Autodesk Inventor part; units mm, degrees
ref_plane "Work Plane1" through (30.1625, 0, 0) normal (0, 0, -1) x (1, 0, 0)
ref_plane "YZ Plane" through (0, 0, 0) normal (1, 0, 0) x (0, 1, 0)
ref_plane "XZ Plane" through (0, 0, 0) normal (0, 1, 0) x (-1, 0, 0)
sketch "Эскиз1" plane through (0, 0, 0) normal (0, 0, 1) x (1, 0, 0)
  line L0 (-6, 0) -> (25, 0)
  line L1 (25, 0) -> (25, 5)
  line L2 (25, 5) -> (1.5, 5)
  line L3 (1.5, 5) -> (0.5798, 5)
  line L4 (0.5798, 5) -> (0, 5)
  line L5 (0, 5) -> (0, 8)
  line L6 (-12.2, 0) -> (31.2, 0)
  line L7 (0, -1.6) -> (0, 9.6)
  line L8 (-6, 0) -> (-6, 8)
  line L9 (0, 8) -> (-6, 8)
  dimension "d0" = 25
  dimension "d1" = 23.5
  dimension "d2" = 0.9202
  dimension "d3" = 6
  dimension "d4" = 10
  dimension "d5" = 10
  dimension "d9" = 16
  dimension "d10" = 0
revolve "Базовый элемент" add sketch "Эскиз1" angle 360 about axis through (-6, 0, 0) along (1, 0, 0)
sketch "Эскиз2" plane through (-6, 0, 0) normal (-1, 0, 0) x (0, 0, 1)
  circle A0 centre (0, 0) radius 8
  line L0 (0, 0) -> (0, 8)
  line L1 (-8, 1.05) -> (8, 1.05)
  line L2 (8, 1.05) -> (8, -1.05)
  line L3 (8, -1.05) -> (-8, -1.05)
  line L4 (-8, -1.05) -> (-8, 1.05)
  line L5 (-8, 0) -> (8, 0) construction
  line L6 (0, 1.05) -> (0, -1.05) construction
  dimension "d11" = 2.1
  dimension "d12" = 16
fillet "Сопряжение1" radius 0.01 1 edges at (-6, -8, 0)
extrude "Паз" cut sketch "Эскиз2" against normal blind 4.2 contours A0 L3 L1 | L2 L3 A0 | A0 L1 L2 | L3 L4 A0 | A0 L4 L1
thread "Резьба"
chamfer "Chamfer4" distance 1 angle 45 1 edges at (25, -5, 0)
ref_plane "Work Plane1" through (30.1625, 0, 0) normal (0, 0, -1) x (1, 0, 0)
equation "\"d11\" = SBR"
equation "\"d12\" = KOD"
equation "\"d13\" = RR"
equation "\"d16\" = STI"
equation "\"d14\" = GEL"
equation "\"d40\" = 0.1 * GD"
equation "\"d0\" = NLG"
equation "\"d1\" = GEL"
equation "\"d2\" = GAL"
equation "\"d3\" = KOH"
equation "\"d4\" = GD"
equation "\"d5\" = BDM"
equation "\"d9\" = KOD"
equation "\"GD\" = NND"
equation "\"NLG\" = 25"
equation "\"GEL\" = 23.5"
equation "\"KOD\" = 16"
equation "\"KOH\" = 6"
equation "\"GAL\" = 0.61345 * PTC"
equation "\"BDM\" = NND"
equation "\"RR\" = 0.01"
equation "\"SBR\" = 2.1"
equation "\"STI\" = 4.2"
equation "\"KEWI\" = 0"
equation "\"GUL\" = 0.61345 * PTC"
equation "\"SPD\" = NND - 1.2269 * PTC"
equation "\"PTC\" = 1.5"
equation "\"TOA\" = 30deg"
equation "\"FAWI\" = 45deg"
equation "\"GD1\" = THREADDIA - 1.2269 * PTC"
properties part number "Винт M10-6gx25 ГОСТ 1491-80" material "Сталь, мягкая"
Here's how the part is built. I have some questions about the finished solid (model axes, mm). A direction names the side the tool comes from. Round coordinates to 2 decimals unless told otherwise and drop trailing zeros. Order: outer loops, then holes, each group sorted by start corner. A loop starts at its lowest first (then second) coordinate and runs counter-clockwise, first axis right, second up. Notation, with made-up numbers: M 17.5,-20 L 48.5,-20 A12 cw 48.5,3 Z; hole C 80,8 d10. An arc over 180 degrees is marked long. Return JSON: item names as keys, results as strings. Group by question number.
1. If we section it at C-C on x = 16: List the corners of the cut face in (y, z) for me.
2. Please list where these lines run through material, in increasing order: probe 1 along X at (y, z) = (-6.5, 4); probe 2 along X at (y, z) = (0.75, -2.5); probe 3 along Y at (x, z) = (18.5, 3).
3. If we section it at A-A on y = 0: List the corners of the cut face in (x, z) for me, then the cut area to 3 significant figures.
4. On a 3-axis mill with a long thin cutter (end or side, diameter ignored), from which of +Z, -Z, +X, -X, +Y, -Y can I reach the whole of each face in a straight line? I mean faces 1 (the face through (0, -0.1, -5.2)), 2 (the face through (-6, -4, 0)), 3 (the face through (-4, -1.05, 0)). Say none if no direction works.
5. I'm going to push flat-ended pins straight in: pin 1 Ø1.3 at (x, z) = (-3.5, -3) entering from +Y; pin 2 Ø3 at (x, z) = (18.5, 3.5) entering from +Y; pin 3 Ø4 at (x, z) = (18.5, 6) entering from -Y. Where does each tip first touch, or does it pass through?
6. If we mould it in two halves opening along Y, with no side actions, what happens to faces 4 (the face through (11.83, -1.08, 4.88)), 5 (the face through (-1.8, 0, 0)), 6 (the face through (25, 0, 0)), 7 (the face through (-4, 1.05, 0))? For each: pulls with the +Y half, pulls with the -Y half, needs draft (parallel to the pull), parting line crosses it, or undercut.
Reply:
{
 "1": {"outline": "C 0,0 d10"},
 "2": {"probe 1": "-6 to 0", "probe 2": "-1.8 to 25", "probe 3": "-4 to 4"},
 "3": {"outline": "M -1.8,-8 L 0,-8 L 0,-5 L 24,-5 L 25,-4 L 25,4 L 24,5 L 0,5 L 0,8 L -1.8,8 Z", "area": "278 mm^2"},
 "4": {"face 1": "+X", "face 2": "+Z, -Z, -X, +Y, -Y", "face 3": "+Z, -Z, -X"},
 "5": {"pin 1": "y = 7.65", "pin 2": "y = 4.58", "pin 3": "y = -3"},
 "6": {"face 4": "parting line crosses it", "face 5": "undercut", "face 6": "needs draft", "face 7": "undercut"}
}
